The listing builds one solid part. Answer for the finished solid, in the listing's coordinates (mm). Face numbers are marked on the shaded views. A direction names the side the tool comes from. Give positions to 0.01 mm unless a question says otherwise; leave off trailing zeros. Loops run counter-clockwise (first coordinate to the right, second up) from the corner with the lowest first, then second, coordinate; pieces in that order, holes last. Notation, with made-up numbers: (40.5, -30) - (99.5, -30) arc R11 ccw to (99.5, -17) - close; hole circle Ø8 at (73, 45.5). An arc over 180 degrees is marked (long way). One line per item, written item: value. Start each with the question number.
from build123d import *

# Parameters (mm, degrees)
SKETCH8_W           = 7
SKETCH8_H           = 7
BOSS_EXTRUDE3_DEPTH = 2
SKETCH9_R           = 2.9
BOSS_EXTRUDE4_DEPTH = 4
SKETCH10_R          = 2.5
SKETCH10_R_2        = 1.25
BOSS_EXTRUDE5_DEPTH = 19
FILLET1_SIZE        = 1


with BuildPart() as part:
    # Sketch8 → Boss-Extrude3 (new body)
    with BuildSketch(Plane(origin=(0, 0, 0), x_dir=(1, 0, 0), z_dir=(0, 1, 0))):
        Rectangle(SKETCH8_W, SKETCH8_H)
    extrude(amount=BOSS_EXTRUDE3_DEPTH)

    # Sketch9 → Boss-Extrude4 (add)
    with BuildSketch(Plane(origin=(0, 2, 0), x_dir=(1, 0, 0), z_dir=(0, 1, 0))):
        with Locations(Location((0, 0, 0), (0, 0, 270))):
            Circle(SKETCH9_R)
    extrude(amount=BOSS_EXTRUDE4_DEPTH)

    # Sketch10 → Boss-Extrude5 (add)
    with BuildSketch(Plane.XZ):
        with Locations(Location((0, 0, 0), (0, 0, 90))):
            Circle(SKETCH10_R)
        with Locations(Location((0, 0, 0), (0, 0, 270))):
            Circle(SKETCH10_R_2, mode=Mode.SUBTRACT)
    extrude(amount=BOSS_EXTRUDE5_DEPTH)

    # Fillet1
    # a fillet whose section is not a circle: 1 mm, written as the material it takes off along each edge
    with BuildSketch(Plane(origin=(0, 6, 0), x_dir=(0, 0, 1), z_dir=(-1, 0, 0))) as fillet1_piece_1:
        with BuildLine():
            add(Edge.make_bspline([(2.9, -FILLET1_SIZE), (2.9, -FILLET1_SIZE * 0.831801948466), (2.9, -FILLET1_SIZE * 0.663603896932), (2.9 - FILLET1_SIZE * 0.0716919198361, -FILLET1_SIZE * 0.292893218813), (2.9 - FILLET1_SIZE * 0.292893218813, -FILLET1_SIZE * 0.0716919198361), (2.9 - FILLET1_SIZE * 0.663603896932, 0), (2.9 - FILLET1_SIZE * 0.831801948466, 0), (2.9 - FILLET1_SIZE, 0)], knots=[0, 0, 0, 0, 0, 0, 0.5, 0.5, 1, 1, 1, 1, 1, 1], degree=5))
            Line((2.9 - FILLET1_SIZE, 0), (2.9, 0))
            Line((2.9, 0), (2.9, -FILLET1_SIZE))
        make_face()
    revolve(axis=Axis((0, 6, 0), (0, 1, 0)), mode=Mode.SUBTRACT)


solid = part.part
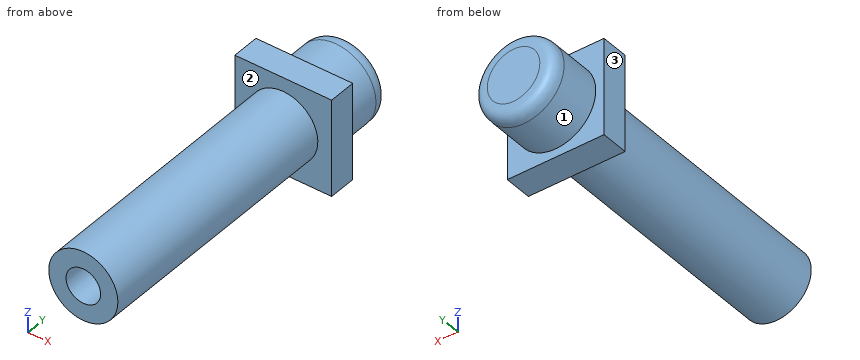
1. For the marked faces 1, 2 and 3, determine the directions among +Z, -Z, +X, -X, +Y, -Y from which every point of the face is accessible in a straight line to the end or side of a thin tool.
2. Find the intervals of material crossed by L1, parallel to X at y = -14.5, z = 0; L2, parallel to Y at x = -2, z = -2.25; L3, parallel to Y at x = 1, z = 0.5, in increasing order. Write a range as [from, to].
3. A cutting plane is placed at A-A (y = -17). Determine the outline of the cut face in (x, z), plus the area to 3 significant figures.
4. A flat-ended cylindrical pin translates along its axis: pin 1 (2 mm diameter, centred on x = 0, z = 0, fed in from -Y). Find the tip coordinate at first contact, or state that the pin passes through.
Results below:
1. face 1: +Y
1. face 2: -Y
1. face 3: +Z, -Z, -X, +Y, -Y
2. L1: x = [-2.5, -1.25], [1.25, 2.5]
2. L2: y = [0, 2]
2. L3: y = [0, 6]
3. outline: circle Ø5 at (0, 0); hole circle Ø2.5 at (0, 0)
3. area: 14.7 mm^2
4. pin 1: stops at y = 0
